```python
from build123d import *

# Parameters (mm, degrees)
SKETCH4_W           = 6.858
SKETCH4_H           = 25.908
SKETCH4_W_2         = 6.5024
SKETCH4_H_2         = 12.8524
BOSS_EXTRUDE1_DEPTH = 6.35
CUT_EXTRUDE1_DEPTH  = 150.225
FILLET1_R           = 2.54
CHAMFER1_SIZE       = 3.175


with BuildPart() as part:
    # Sketch4 → Boss-Extrude1 (new body)
    with BuildSketch(Plane(origin=(0, 0, 0), x_dir=(0, 0, -1), z_dir=(1, 0, 0))):
        Polygon((0, 6.35), (-60.325, 6.35), (-60.325, 32.004), (-60.325, 44.704), (-60.325, 133.35), (66.675, 133.35), (66.675, 44.704), (66.675, 32.004), (66.675, 6.35), (6.35, 6.35), (6.35, 0), (0, 0), align=None)
        with Locations((3.175, 95.25)):
            Rectangle(SKETCH4_W, SKETCH4_H, mode=Mode.SUBTRACT)
        with Locations((-50.8, 38.1)):
            Rectangle(SKETCH4_W_2, SKETCH4_H_2, mode=Mode.SUBTRACT)
        with Locations((57.15, 38.1)):
            Rectangle(SKETCH4_W_2, SKETCH4_H_2, mode=Mode.SUBTRACT)
    extrude(amount=BOSS_EXTRUDE1_DEPTH)

    # Sketch5 → Cut-Extrude1 (cut, through all)
    with BuildSketch(Plane(origin=(6.35, 0, 0), x_dir=(0, 0, -1), z_dir=(1, 0, 0))):
        Polygon((-28.836084591, 61.9125), (-44.45, 99.646128904), (-44.45, 24.178871096), align=None)
        Polygon((-9.786084591, 107.95), (-41.013915409, 107.95), (-25.4, 70.216371096), align=None)
        Polygon((-9.786084591, 15.875), (-25.4, 53.608628904), (-41.013915409, 15.875), align=None)
        Polygon((28.313915409, 61.9125), (12.7, 99.646128904), (12.7, 24.178871096), align=None)
        Polygon((47.363915409, 107.95), (16.136084591, 107.95), (31.75, 70.216371096), align=None)
        Polygon((50.8, 99.646128904), (35.186084591, 61.9125), (50.8, 24.178871096), align=None)
        Polygon((47.363915409, 15.875), (31.75, 53.608628904), (16.136084591, 15.875), align=None)
        Polygon((-6.35, 99.646128904), (-21.963915409, 61.9125), (-6.35, 24.178871096), align=None)
    extrude(amount=-CUT_EXTRUDE1_DEPTH, mode=Mode.SUBTRACT)

    # Fillet1
    fillet1_edges = [part.edges().sort_by_distance(p)[0] for p in [
        (3.175, 53.608628904, 25.4),
        (3.175, 15.875, 9.786084591),
        (3.175, 70.216371096, -31.75),
        (3.175, 107.95, -16.136084591),
        (3.175, 107.95, -47.363915409),
        (3.175, 61.9125, -28.313915409),
        (3.175, 24.178871096, -12.7),
        (3.175, 99.646128904, -12.7),
        (3.175, 15.875, -47.363915409),
        (3.175, 15.875, -16.136084591),
        (3.175, 53.608628904, -31.75),
        (3.175, 24.178871096, -50.8),
        (3.175, 61.9125, -35.186084591),
        (3.175, 99.646128904, -50.8),
        (3.175, 61.9125, 21.963915409),
        (3.175, 99.646128904, 6.35),
        (3.175, 24.178871096, 6.35),
        (3.175, 24.178871096, 44.45),
        (3.175, 99.646128904, 44.45),
        (3.175, 61.9125, 28.836084591),
        (3.175, 70.216371096, 25.4),
        (3.175, 107.95, 41.013915409),
        (3.175, 107.95, 9.786084591),
        (3.175, 15.875, 41.013915409),
    ]]
    fillet(fillet1_edges, radius=FILLET1_R)

    # Chamfer1
    chamfer1_edges = [part.edges().sort_by_distance(p)[0] for p in [
        (0, 133.35, -3.175),
    ]]
    chamfer(chamfer1_edges, length=CHAMFER1_SIZE)


solid = part.part
```
The listing builds one solid part. Answer for the finished solid, in the listing's coordinates (mm). A direction names the side the tool comes from. Coordinates: 2 decimals unless noted, no trailing zeros. Loops run counter-clockwise (first coordinate to the right, second up) from the corner with the lowest first, then second, coordinate; pieces in that order, holes last. Notation, with made-up numbers: M -27,14 L -20,14 A23 cw -20,48 Z; hole C 26,27 d10. An arc over 180 degrees is marked long. Answer as a JSON object with one key per item and string values. Group by question number.
Item 1: Consider L1, parallel to Y at x = 3, z = -32 (3 decimals); L2, parallel to Z at x = 2, y = 26 (3 decimals); L3, parallel to Z at x = 5.5, y = 68.5 (3 decimals). Determine where each line is inside the solid, lowest interval first.
Item 2: Section D-D (y = 79) is taken. Write down the section's boundary in (x, z) (3 decimals), and give its area (3 significant figures).
Item 3: Determine the mould class of faces 1 (the face through (3, 6.35, -37)), 2 (the face through (3.131, 49.505, 25.358)), 3 (the face through (3, 3, -6.35)) for opening direction Z: +Z half, -Z half, draft (parallel to the pull), parting line (faces both ways), or undercut.
Item 4: Section B-B (y = 54) is taken. Write down the section's boundary in (x, z) (3 decimals).
Item 5: Section A-A (z = -4) is taken. Write down the section's boundary in (x, y) (3 decimals), and give its area (3 significant figures).
Item 6: Section C-C (z = 25.5) is taken. Write down the section's boundary in (x, y) (3 decimals).
Item 7: Each of these flat-tipped pins is pushed along its axis until it touches: P1, Ø1.9, axis at x = 2.5, z = -1.5, coming from the -Y side; P2, Ø3, axis at x = 4.5, y = 2, coming from the -Z side; P3, Ø1, axis at x = 1.5, z = -34, coming from the +Y side (3 decimals); P4, Ø3, axis at x = 1.5, z = -3.5, coming from the +Y side (3 decimals). Where does it stop, or does it pass through?
Item 8: Which of the six approach directions +Z, -Z, +X, -X, +Y, -Y give full straight-line access (tool end or side, diameter ignored) to faces 4 (the face through (6.35, 68, -4)), 5 (the face through (3.22, 75.53, 16.33))?
Solved:
{
 "1": {"L1": "y = 6.35 to 15.875, 49.493 to 74.332, 107.95 to 133.175", "L2": "z = -66.675 to -43.174, -20.326 to 13.976, 36.824 to 60.325", "L3": "z = -66.675 to -50.8, -37.912 to -25.588, -12.7 to 6.35, 19.238 to 31.562, 44.45 to 60.325"},
 "2": {"outline": "M 0,-66.675 L 6.35,-66.675 L 6.35,-50.8 L 0,-50.8 Z; M 0,-42.257 L 6.35,-42.257 L 6.35,-35.385 L 0,-35.385 Z; M 0,-28.115 L 6.35,-28.115 L 6.35,-21.243 L 0,-21.243 Z; M 0,-12.7 L 6.35,-12.7 L 6.35,6.35 L 0,6.35 Z; M 0,14.893 L 6.35,14.893 L 6.35,21.765 L 0,21.765 Z; M 0,29.035 L 6.35,29.035 L 6.35,35.907 L 0,35.907 Z; M 0,44.45 L 6.35,44.45 L 6.35,60.325 L 0,60.325 Z", "area": "497 mm2"},
 "3": {"face 1": "draft", "face 2": "undercut", "face 3": "-Z half"},
 "4": {"outline": "M 0,-66.675 L 6.35,-66.675 L 6.35,-50.8 L 0,-50.8 Z; M 0,-38.46 L 6.35,-38.46 L 6.35,-25.04 L 0,-25.04 Z; M 0,-12.7 L 6.35,-12.7 L 6.35,6.35 L 0,6.35 Z; M 0,18.69 L 6.35,18.69 L 6.35,32.11 L 0,32.11 Z; M 0,44.45 L 6.35,44.45 L 6.35,60.325 L 0,60.325 Z"},
 "5": {"outline": "M 0,0 L 6.35,0 L 6.35,82.296 L 0,82.296 Z; M 0,108.204 L 6.35,108.204 L 6.35,133.35 L 3.175,133.35 L 0,130.175 Z", "area": "677 mm2"},
 "6": {"outline": "M 0,6.35 L 6.35,6.35 L 6.35,15.875 L 0,15.875 Z; M 0,49.504 L 6.35,49.504 L 6.35,74.321 L 0,74.321 Z; M 0,107.95 L 6.35,107.95 L 6.35,133.35 L 3.175,133.35 L 0,130.175 Z"},
 "7": {"P1": "stops at y = 0", "P2": "stops at z = -6.35", "P3": "stops at y = 132.175", "P4": "stops at y = 133.175"},
 "8": {"face 4": "+Z, -Z, +X, +Y, -Y", "face 5": "+X, -X"}
}
